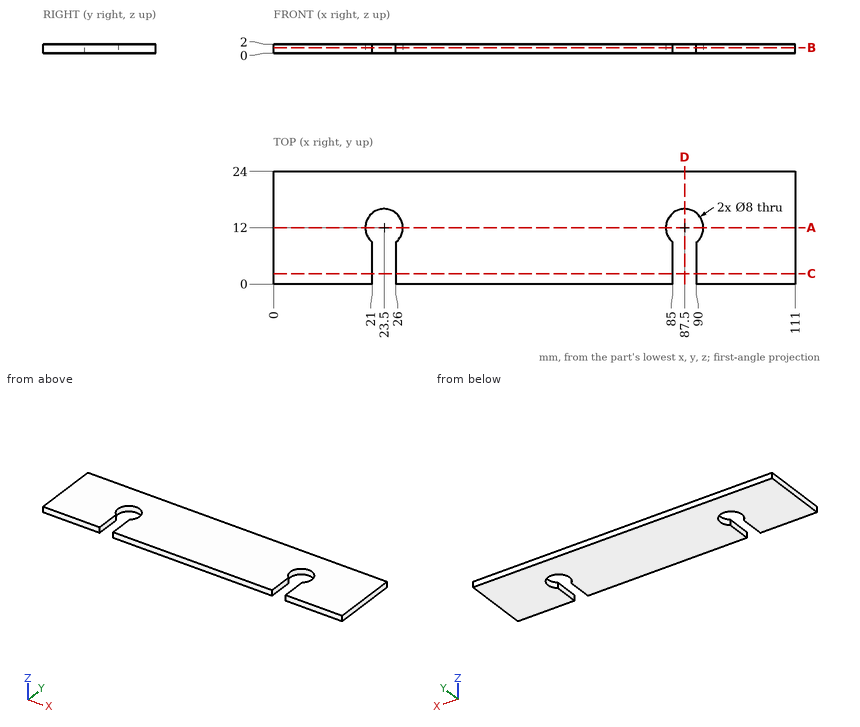
The figure shows three views and two pictorial views of one solid part (mm, origin at its lowest corner). Answer the questions. Round coordinates to 2 decimals unless told otherwise and drop trailing zeros. Order: outer loops, then holes, each group sorted by start corner. A loop starts at its lowest first (then second) coordinate and runs counter-clockwise, first axis right, second up. Notation, with made-up numbers: M 71,52 L 121,52 A16 cw 121,63 Z; hole C 12,62 d9. An arc over 180 degrees is marked long. Put each result on its own line as item: value. Start each with the question number.
Q1. Section B-B, the plane z = 1.25 is taken. Write down the section's boundary in (x, y).
Q2. Straight lines are drawn through the part: L1, parallel to X at y = 12, z = 0.7; L2, parallel to X at y = 6.5, z = 1.3; L3, parallel to Y at x = 87.5, z = 1.5. For each, find the intervals that lie inside material, in ascending order. Write a range as [from, to].
Q3. Section D-D, the plane x = 87.5 is taken. Write down the section's boundary in (y, z), and give its area (3 significant figures).
Q4. Section A-A, the plane y = 12 is taken. Write down the section's boundary in (x, z).
Q5. Section C-C, the plane y = 2.25 is taken. Write down the section's boundary in (x, z).
Findings below:
1. outline: M 0,0 L 21,0 L 21,8.88 A4 cw long 26,8.88 L 26,0 L 85,0 L 85,8.88 A4 cw long 90,8.88 L 90,0 L 111,0 L 111,24 L 0,24 Z
2. L1: x = [0, 19.5], [27.5, 83.5], [91.5, 111]
2. L2: x = [0, 21], [26, 85], [90, 111]
2. L3: y = [16, 24]
3. outline: M 16,0 L 24,0 L 24,2 L 16,2 Z
3. area: 16.0 mm^2
4. outline: M 0,0 L 19.5,0 L 19.5,2 L 0,2 Z; M 27.5,0 L 83.5,0 L 83.5,2 L 27.5,2 Z; M 91.5,0 L 111,0 L 111,2 L 91.5,2 Z
5. outline: M 0,0 L 21,0 L 21,2 L 0,2 Z; M 26,0 L 85,0 L 85,2 L 26,2 Z; M 90,0 L 111,0 L 111,2 L 90,2 Z
